from build123d import *

# Parameters (mm, degrees)
SCHIZZO1_R                    = 16.5
SCHIZZO1_R_2                  = 14
SCHIZZO1_R_3                  = 12
SCHIZZO1_R_4                  = 9.5
ESTRUSIONE_ESTRUSIONE1_DEPTH  = 1.5
ESTRUSIONE_SOTTILE4_DEPTH     = 15
ESTRUSIONE_ESTRUSIONE2_DEPTH  = 25
TAGLIO_ESTRUSIONE1_DEPTH      = 23.5
TAGLIO_ESTRUSIONE2_DEPTH      = 214.121208684
TAGLIO_ESTRUSIONE2_DEPTH_BACK = 214.121208684
ESTRUSIONE_SOTTILE5_DEPTH     = 15
ESTRUSIONE_ESTRUSIONE3_DEPTH  = 1.5
TAGLIO_ESTRUSIONE4_START      = -4.28444402
TAGLIO_ESTRUSIONE4_DEPTH      = 61.768658905
ESTRUSIONE_ESTRUSIONE5_DEPTH  = 2
RACCORDO4_R                   = 3
RACCORDO5_R                   = 3


# Read off the part's stored shape, not the designer's step: Taglio-Estrusione4
with BuildPart() as part:
    # Schizzo1 → Estrusione-Estrusione1 (new, symmetric)
    with BuildSketch(Plane.XY):
        Polygon((0, 55), (0, 0), (155, 56.415386311), (155, 84.415386311), align=None)
        with Locations((28.912269587, 35.505040119)):
            Circle(SCHIZZO1_R, mode=Mode.SUBTRACT)
        with Locations((65.534477731, 45.644757604)):
            Circle(SCHIZZO1_R_2, mode=Mode.SUBTRACT)
        with Locations((97.337974277, 54.450301735)):
            Circle(SCHIZZO1_R_3, mode=Mode.SUBTRACT)
        with Locations((123.359016906, 61.654837842)):
            Circle(SCHIZZO1_R_4, mode=Mode.SUBTRACT)
    extrude(amount=ESTRUSIONE_ESTRUSIONE1_DEPTH, both=True)

    # Schizzo5 → Estrusione-Sottile4 (add, symmetric)
    with BuildSketch(Plane.XY):
        Polygon((158, 88.038261311), (-3, 57.484214885), (-3, -4.28444402), (158, 54.314763697), align=None)
        Polygon((155, 84.415386311), (0, 55), (0, 0), (155, 56.415386311), align=None, mode=Mode.SUBTRACT)
    extrude(amount=ESTRUSIONE_SOTTILE4_DEPTH, both=True)

    # Schizzo6 → Estrusione-Estrusione2 (add, symmetric)
    with BuildSketch(Plane.XY):
        with BuildLine():
            Line((143.08944618, 67.455418384), (148.573566634, 112.119995208))
            ThreePointArc((148.573566634, 112.119995208), (161.946552574, 122.568116907), (172.394674273, 109.195130967))
            Line((172.394674273, 109.195130967), (166.91055382, 64.530554143))
            ThreePointArc((166.91055382, 64.530554143), (153.537567879, 54.082432444), (143.08944618, 67.455418384))
        make_face()
    extrude(amount=ESTRUSIONE_ESTRUSIONE2_DEPTH, both=True)

    # Schizzo7 → Taglio-Estrusione1 (cut)
    with BuildSketch(Plane.XY.offset(25)):
        with BuildLine():
            Line((163.932915365, 64.896162173), (169.417035818, 109.560738997))
            ThreePointArc((169.417035818, 109.560738997), (161.580944544, 119.590478452), (151.551205088, 111.754387178))
            Line((151.551205088, 111.754387178), (146.067084635, 67.089810354))
            ThreePointArc((146.067084635, 67.089810354), (153.903175909, 57.060070899), (163.932915365, 64.896162173))
        make_face()
    taglio_estrusione1 = extrude(amount=-TAGLIO_ESTRUSIONE1_DEPTH, mode=Mode.SUBTRACT)

    # Specchia1: Taglio-Estrusione1 across plane
    add(taglio_estrusione1.mirror(Plane.XY), mode=Mode.SUBTRACT)

    # Schizzo8 → Taglio-Estrusione2 (cut, two sides: drawn at the far end of the back side and taken through both)
    with BuildSketch(Plane.XY.offset(-TAGLIO_ESTRUSIONE2_DEPTH_BACK)):
        with BuildLine():
            Line((149.088066357, 75.282713956), (152.500407973, 103.074006202))
            ThreePointArc((152.500407973, 103.074006202), (160.301316438, 109.16874386), (166.396054096, 101.367835395))
            Line((166.396054096, 101.367835395), (162.98371248, 73.576543149))
            ThreePointArc((162.98371248, 73.576543149), (155.182804015, 67.481805491), (149.088066357, 75.282713956))
        make_face()
    extrude(amount=TAGLIO_ESTRUSIONE2_DEPTH + TAGLIO_ESTRUSIONE2_DEPTH_BACK, mode=Mode.SUBTRACT)

    # Schizzo9 → Estrusione-Sottile5 (add, symmetric)
    with BuildSketch(Plane.XY):
        Polygon((-3, 57.484214885), (-20, 54.258011225), (-20, -4.28444402), (-17, -4.28444402), (-17, 51.77379634), (-2.440653337, 54.536820898), align=None)
    extrude(amount=ESTRUSIONE_SOTTILE5_DEPTH, both=True)

    # Schizzo12 → Estrusione-Estrusione3 (add, symmetric)
    with BuildSketch(Plane.XY):
        Polygon((-17, 51.77379634), (-17, -4.28444402), (-3, -4.28444402), (-3, 54.430669942), align=None)
    extrude(amount=ESTRUSIONE_ESTRUSIONE3_DEPTH, both=True)

    # Taglio-Estrusione4 outline → Taglio-Estrusione4 (cut)
    with BuildSketch(Plane(origin=(0, 0, 0), x_dir=(1, 0, 0), z_dir=(0, 1, 0)).offset(TAGLIO_ESTRUSIONE4_START)):
        Polygon((-3, -15), (-17, -10), (-20, -10), (-20, -15), align=None)
    extrude(amount=TAGLIO_ESTRUSIONE4_DEPTH, mode=Mode.SUBTRACT)

    # Schizzo22 → Estrusione-Estrusione5 (add, symmetric)
    with BuildSketch(Plane.XY):
        with BuildLine():
            Line((-19, -4.28444402), (-19, -11.077337239))
            ThreePointArc((-19, -11.077337239), (-18.691341716, -11.539277005), (-18.146446609, -11.43089063))
            Line((-18.146446609, -11.43089063), (-15, -8.28444402))
            Line((-15, -8.28444402), (-17, -8.28444402))
            Line((-17, -8.28444402), (-17, -4.28444402))
            Line((-17, -4.28444402), (-19, -4.28444402))
        make_face()
    extrude(amount=ESTRUSIONE_ESTRUSIONE5_DEPTH, both=True)

    # Raccordo4
    raccordo4_edges = [part.edges().sort_by_distance(p)[0] for p in [
        (153.537567879, 54.082432444, 25),
        (169.652614046, 86.862842555, 25),
        (161.946552574, 122.568116907, 25),
        (145.831506407, 89.787706796, 25),
    ]]
    fillet(raccordo4_edges, radius=RACCORDO4_R - 0.0001)  # a hair under: the kernel refuses the full size

    # Raccordo5
    raccordo5_edges = [part.edges().sort_by_distance(p)[0] for p in [
        (145.831506407, 89.787706796, -25),
        (153.537567879, 54.082432444, -25),
        (169.652614046, 86.862842555, -25),
        (161.946552574, 122.568116907, -25),
    ]]
    fillet(raccordo5_edges, radius=RACCORDO5_R - 0.0001)  # a hair under: the kernel refuses the full size


solid = part.part
Build history of the part. All positions in model axes, mm. A direction names the side the tool comes from. Give positions to 0.01 mm unless a question says otherwise; leave off trailing zeros. Loops run counter-clockwise (first coordinate to the right, second up) from the corner with the lowest first, then second, coordinate; pieces in that order, holes last. Notation, with made-up numbers: (65, 75) -> (119, 75) arc R34 cw to (119, 106) -> close; hole circle Ø2 at (29.5, 36). An arc over 180 degrees is marked (long way). Answer in a Markdown table with one row per item.
Item 1: Flat gauge pins, fed straight in: P1, Ø3, axis at y = 90.5, z = 17, coming from the -X side; P2, Ø12, axis at x = 130.5, z = 13, coming from the -Y side; P3, Ø3, axis at y = -9, z = -0.5, coming from the -X side. Where does each tip first touch, or does it go through?
Findings below:
| item | result |
|---|---|
| P1 | stops at x = 145.73 |
| P2 | stops at y = 42.12 |
| P3 | stops at x = -19 |
Item 2: Tool access for faces 1 (the flat face through (73.483, 68.945, 8.344)), 2 (the flat face through (-18, -8, 2)), 3 (the flat face through (74.26, 27.03, -8.16)): list every direction of +Z, -Z, +X, -X, +Y, -Y with a clear straight run to the whole face (end or side of a thin tool).
Findings below:
| item | result |
|---|---|
| face 1 | +Z |
| face 2 | +Z, +X, -X, -Y |
| face 3 | -Z |
Item 3: Slice it at B-B on y = 29. Write the cut outline in (x, z), plus the area to 3 significant figures.
Findings below:
| item | result |
|---|---|
| outline | (-20, -15) -> (-17, -15) -> (-17, -1.5) -> (-3, -1.5) -> (-3, -15) -> (0, -15) -> (0, -1.5) -> (13.75, -1.5) -> (13.75, 1.5) -> (0, 1.5) -> (0, 15) -> (-3, 15) -> (-3, 1.5) -> (-17, 1.5) -> (-17, 10) -> (-20, 10) -> close; (44.08, -1.5) -> (79.68, -1.5) -> (79.68, -15) -> (88.45, -15) -> (88.45, 15) -> (79.68, 15) -> (79.68, 1.5) -> (44.08, 1.5) -> close |
| area | 618 mm² |
Item 4: Mould opens along X. For faces 4 (the flat face through (-18, -8, -2)), 5 (the flat face through (73.483, 68.945, -8.156)), 6 (the flat face through (76.373, 24.605, 0.21)) say: pulls with the +X half, pulls with the -X half, needs draft (parallel to the pull), parting line crosses it, or undercut.
Findings below:
| item | result |
|---|---|
| face 4 | needs draft |
| face 5 | undercut |
| face 6 | pulls with the +X half |
Item 5: Slice it at A-A on z = 7.5. Write the cut outline in (x, y), plus the area to 3 significant figures.
Findings below:
| item | result |
|---|---|
| outline | (-20, -4.28) -> (-17, -4.28) -> (-17, 51.77) -> (-3, 54.43) -> (-3, -4.28) -> (158, 54.31) -> (158, 54.37) arc R12 ccw to (166.91, 64.53) -> (172.39, 109.2) arc R12 ccw to (148.57, 112.12) -> (145.32, 85.63) -> (-20, 54.26) -> close; hole (0, 0) -> (150.62, 54.82) arc R12 cw to (143.09, 67.46) -> (144.94, 82.51) -> (0, 55) -> close; hole (146.07, 67.09) arc R9 ccw to (163.93, 64.9) -> (169.42, 109.56) arc R9 ccw to (151.55, 111.75) -> close |
| area | 1,800 mm² |
Item 6: Slice it at C-C on x = 22.5. Write the cut outline in (y, z).
Findings below:
| item | result |
|---|---|
| outline | (5, -15) -> (8.19, -15) -> (8.19, -1.5) -> (20.3, -1.5) -> (20.3, 1.5) -> (8.19, 1.5) -> (8.19, 15) -> (5, 15) -> close; (50.71, -1.5) -> (59.27, -1.5) -> (59.27, -15) -> (62.32, -15) -> (62.32, 15) -> (59.27, 15) -> (59.27, 1.5) -> (50.71, 1.5) -> close |
Item 7: Probe line 1 along Z through (x, y) = (-10, 24); line 2 along X through (y, z) = (73.5, -22.5); line 3 along X through (y, z) = (74, 22.5). List the from-to ranges inside material, lowest first. Write a range as [from, to].
Findings below:
| item | result |
|---|---|
| line 1 | z = [-1.5, 1.5] |
| line 2 | x = [143.87, 146.85], [164.99, 167.97] |
| line 3 | x = [143.94, 146.92], [165.05, 168.03] |
